Input: dimensioned drawing with shaded views. Units: mm. Origin: part minimum x, y, z. A direction names the side the tool comes from. Coordinates: 2 decimals unless noted, no trailing zeros. Order: outer loops, then holes, each group sorted by start corner. A loop starts at its lowest first (then second) coordinate and runs counter-clockwise, first axis right, second up. Notation, with made-up numbers: (86.5, 3.5) - (94.5, 3.5) arc R5 ccw to (94.5, 12.5) - close; hole circle Ø1 at (54.5, 18.25). An arc over 180 degrees is marked (long way). One line per question, with ' | ' between items. Start each with the question number.
(1) Section A-A (z = 16). Return the cut outline in (x, y), then the cut area to 3 significant figures.
(2) Contact query for flat-ended pins moving along their axis: P1, Ø3, axis at y = 26.5, z = 29, coming from the -X side; P2, Ø5, axis at x = 61.5, z = 27, coming from the +Y side (1 decimal); P3, Ø4, axis at x = 30.81, y = 9.19, coming from the +Z side. Output: stop coordinate, or through.
(3) Access query for the marked faces 1, 2 and 3. Directions: +Z, -Z, +X, -X, +Y, -Y. A direction counts if a zero-diameter tool reaches every point of the face in a straight line with its end or side. Return the directions, or none.
(4) Section C-C (x = 40). Return the cut outline in (y, z).
(5) Line query: line 1 along X through (y, z) = (7, 20) (1 decimal); line 2 along Y through (x, z) = (10, 27); line 3 along X through (y, z) = (16.5, 27) (1 decimal). Output: solid intervals per line, ascending.
(6) Section D-D (y = 17.5). Return the cut outline in (x, z).
(7) Section B-B (y = 5.5). Return the cut outline in (x, z).
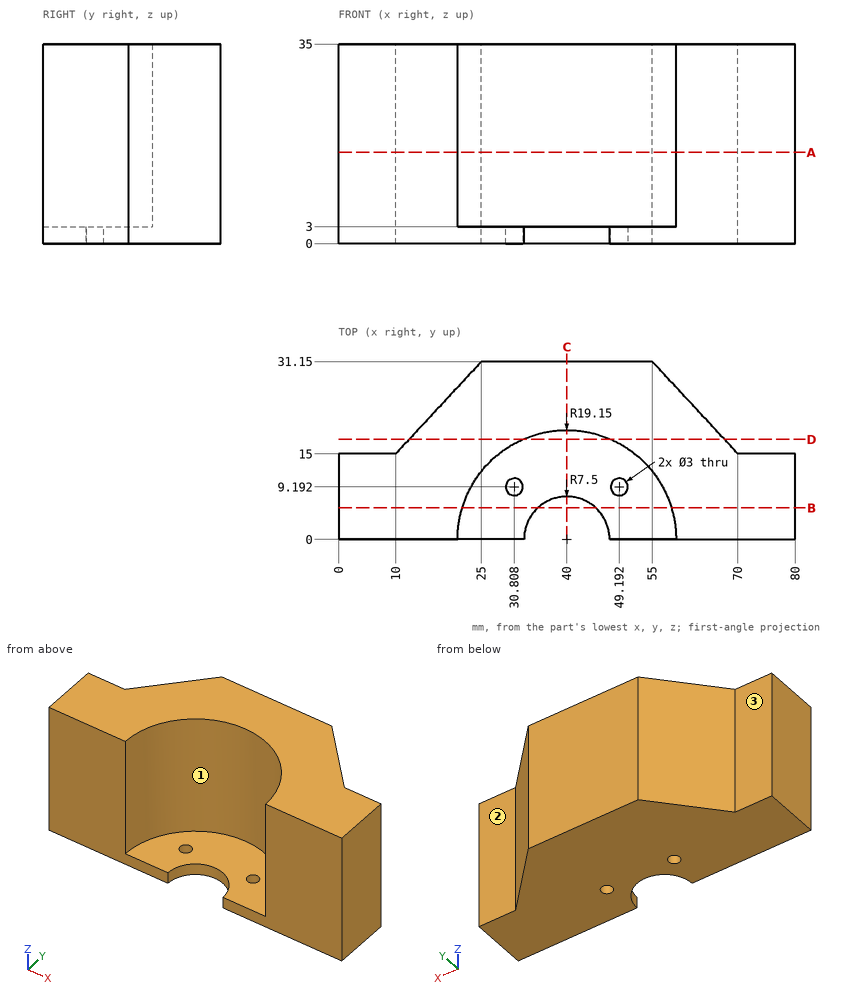
Response values:
1) outline: (0, 0) - (20.85, 0) arc R19.15 cw to (59.15, 0) - (80, 0) - (80, 15) - (70, 15) - (55, 31.15) - (25, 31.15) - (10, 15) - (0, 15) - close | area: 1,350 mm²
2) P1: stops at x = 19.29 | P2: stops at y = 26.8 | P3: stops at z = 3
3) face 1: +Z, -Y | face 2: +Z, -Z, +X, +Y | face 3: +Z, -Z, -X, +Y
4) outline: (7.5, 0) - (31.15, 0) - (31.15, 35) - (19.15, 35) - (19.15, 3) - (7.5, 3) - close
5) line 1: x = 0 to 22.2, 57.8 to 80 | line 2: y = 0 to 15 | line 3: x = 11.4 to 30.3, 49.7 to 68.6
6) outline: (12.32, 0) - (67.68, 0) - (67.68, 35) - (47.78, 35) - (47.78, 3) - (32.22, 3) - (32.22, 35) - (12.32, 35) - close
7) outline: (0, 0) - (34.9, 0) - (34.9, 3) - (21.66, 3) - (21.66, 35) - (0, 35) - close; (45.1, 0) - (80, 0) - (80, 35) - (58.34, 35) - (58.34, 3) - (45.1, 3) - close
